```python
from build123d import *

# Parameters (mm, degrees)
SKETCH1_R           = 17.5
BOSS_EXTRUDE1_DEPTH = 6
SKETCH3_R           = 9
BOSS_EXTRUDE2_DEPTH = 3
CUT_EXTRUDE1_DEPTH  = 10
SKETCH5_R           = 3.5
CUT_EXTRUDE2_DEPTH  = 10


with BuildPart() as part:
    # Sketch1 → Boss-Extrude1 (new body)
    with BuildSketch(Plane(origin=(0, 0, 0), x_dir=(1, 0, 0), z_dir=(0, 1, 0))):
        Circle(SKETCH1_R)
    extrude(amount=BOSS_EXTRUDE1_DEPTH)

    # Sketch3 → Boss-Extrude2 (add)
    with BuildSketch(Plane(origin=(0, 6, 0), x_dir=(1, 0, 0), z_dir=(0, 1, 0))):
        Circle(SKETCH3_R)
    extrude(amount=BOSS_EXTRUDE2_DEPTH)

    # Sketch4 → Cut-Extrude1 (cut, through all)
    with BuildSketch(Plane(origin=(0, 9, 0), x_dir=(1, 0, 0), z_dir=(0, 1, 0))):
        with BuildLine():
            Line((2.667, -1.83711547), (2.667, 1.83711547))
            ThreePointArc((2.667, 1.83711547), (-3.2385, 0), (2.667, -1.83711547))
        make_face()
    extrude(amount=-CUT_EXTRUDE1_DEPTH, mode=Mode.SUBTRACT)

    # Sketch5 → Cut-Extrude2 (cut, through all)
    with BuildSketch(Plane(origin=(0, 0, 0), x_dir=(1, 0, 0), z_dir=(0, 1, 0))):
        with Locations((0, -12.5)):
            Circle(SKETCH5_R)
    extrude(amount=CUT_EXTRUDE2_DEPTH, mode=Mode.SUBTRACT)


solid = part.part
```
Input: part model. Units: mm. Frame: model coordinates. A direction names the side the tool comes from. Give positions to 0.01 mm unless a question says otherwise; leave off trailing zeros. Order: outer loops, then holes, each group sorted by start corner. A loop starts at its lowest first (then second) coordinate and runs counter-clockwise, first axis right, second up. Notation, with made-up numbers: (-10.5, 71) - (14.5, 71) arc R18 ccw to (14.5, 101) - close; hole circle Ø9 at (-3, 24.5). An arc over 180 degrees is marked (long way). Use a Markdown table: item, result.
(1) Pin query (flat end, axial travel): pin 1 (4 mm diameter, centred on y = 6.5, z = -0.5, fed in from -X); pin 2 (1 mm diameter, centred on x = -12, z = 6.5, fed in from +Y); pin 3 (4 mm diameter, centred on x = 0, z = 12.5, fed in from -Y). Return the tip coordinate at first contact, or that it passes through.
Computed values:
| item | result |
|---|---|
| pin 1 | stops at x = -17.5 |
| pin 2 | stops at y = 6 |
| pin 3 | passes through |
(2) Line query: line 1 (Z direction, x = 0, y = 4.75); line 2 (X direction, y = 7, z = 0); line 3 (Z direction, x = 2, y = 0.5). Output: solid intervals per line, ascending. Write a range as from..to.
Computed values:
| item | result |
|---|---|
| line 1 | z = -17.5..-3.24, 3.24..9, 16..17.5 |
| line 2 | x = -9..-3.24, 2.67..9 |
| line 3 | z = -17.39..-2.55, 2.55..9.63, 15.37..17.39 |
(3) Access query for faces 4 (the flat face through (2.667, 5, 0)), 5 (the flat face through (8, 6, -8)), 6 (the flat face through (0, 9, 4)). Directions: +Z, -Z, +X, -X, +Y, -Y. A direction counts if a zero-diameter tool reaches every point of the face in a straight line with its end or side. Return the directions, or none.
Computed values:
| item | result |
|---|---|
| face 4 | +Y, -Y |
| face 5 | +Y |
| face 6 | +Z, -Z, +X, -X, +Y |
(4) Section query B-B (x = -2). Output: boundary loops of the cut face in (y, z).
Computed values:
| item | result |
|---|---|
| outline | (0, -17.39) - (6, -17.39) - (6, -8.77) - (9, -8.77) - (9, -2.55) - (0, -2.55) - close; (0, 2.55) - (9, 2.55) - (9, 8.77) - (6, 8.77) - (6, 9.63) - (0, 9.63) - close; (0, 15.37) - (6, 15.37) - (6, 17.39) - (0, 17.39) - close |
(5) Section query A-A (z = 0). Output: boundary loops of the cut face in (x, y).
Computed values:
| item | result |
|---|---|
| outline | (-17.5, 0) - (-3.24, 0) - (-3.24, 9) - (-9, 9) - (-9, 6) - (-17.5, 6) - close; (2.67, 0) - (17.5, 0) - (17.5, 6) - (9, 6) - (9, 9) - (2.67, 9) - close |
(6) Draft query along X for faces 1 (the cylindrical face through (-3.236, 4.563, -0.115)), 2 (the cylindrical face through (-1.172, 7.479, -8.923)), 3 (the flat face through (4, 0, 0)). Return one class per face: released by +X, released by -X, zero draft, split by the parting line, or undercut.
Computed values:
| item | result |
|---|---|
| face 1 | undercut |
| face 2 | split by the parting line |
| face 3 | zero draft |
(7) Section query D-D (z = -7). Output: boundary loops of the cut face in (x, y), then the cut area to 3 significant figures.
Computed values:
| item | result |
|---|---|
| outline | (-16.04, 0) - (16.04, 0) - (16.04, 6) - (5.66, 6) - (5.66, 9) - (-5.66, 9) - (-5.66, 6) - (-16.04, 6) - close |
| area | 226 mm2 |
(8) Section query C-C (y = 2.5). Output: boundary loops of the cut face in (x, z), then the cut area to 3 significant figures.
Computed values:
| item | result |
|---|---|
| outline | circle Ø35 at (0, 0); hole circle Ø7 at (0, 12.5); hole (2.67, -1.84) - (2.67, 1.84) arc R3.24 ccw (long way) to start |
| area | 892 mm2 |
